from build123d import *

# Parameters (mm, degrees)
SKETCH_1_R      = 2.5
SKETCH_1_R_2    = 12.875
SKETCH_1_R_3    = 13.5
SKETCH_1_R_4    = 2
EXTRUDE_1_DEPTH = 5


with BuildPart() as part:
    # 草圖1 → 填料-伸長1 (new body)
    with BuildSketch(Plane.XY):
        with BuildLine():
            Line((-177.402767175, 46.597232825), (172.597232825, 46.597232825))
            Line((172.597232825, 46.597232825), (172.597232825, -3.218275341))
            Line((172.597232825, -3.218275341), (172.597232825, -12.212255112))
            ThreePointArc((172.597232825, -12.212255112), (171.299816564, -17.138210478), (167.744225572, -20.785962926))
            Line((167.744225572, -20.785962926), (157.766802923, -26.775637768))
            ThreePointArc((157.766802923, -26.775637768), (155.290289709, -27.838762374), (152.619810177, -28.201929955))
            Line((152.619810177, -28.201929955), (-158.204749101, -28.201929955))
            ThreePointArc((-158.204749101, -28.201929955), (-160.839127997, -27.848693549), (-163.287395186, -26.813939522))
            Line((-163.287395186, -26.813939522), (-172.48541326, -21.385442237))
            ThreePointArc((-172.48541326, -21.385442237), (-176.08684631, -17.731937443), (-177.402767175, -12.77343267))
            Line((-177.402767175, -12.77343267), (-177.402767175, -10.307650594))
            Line((-177.402767175, -10.307650594), (-177.402767175, -3.218275341))
            Line((-177.402767175, -3.218275341), (-177.402767175, 46.597232825))
        make_face()
        with Locations((118.590211239, 1.636058568)):
            Circle(SKETCH_1_R, mode=Mode.SUBTRACT)
        with Locations((154.590211239, 1.636058568)):
            Circle(SKETCH_1_R, mode=Mode.SUBTRACT)
        with Locations((136.590211239, 1.636058568)):
            Circle(SKETCH_1_R_2, mode=Mode.SUBTRACT)
        with Locations((-143.364629919, 1.616144457)):
            Circle(SKETCH_1_R_3, mode=Mode.SUBTRACT)
        with Locations((-130.636707858, 14.344066518)):
            Circle(SKETCH_1_R, mode=Mode.SUBTRACT)
        with Locations((-156.09255198, 14.344066518)):
            Circle(SKETCH_1_R, mode=Mode.SUBTRACT)
        with Locations((-130.636707858, -11.111777604)):
            Circle(SKETCH_1_R, mode=Mode.SUBTRACT)
        with Locations((-156.09255198, -11.111777604)):
            Circle(SKETCH_1_R, mode=Mode.SUBTRACT)
        with Locations((-152.402767175, 36.597232825)):
            Circle(SKETCH_1_R, mode=Mode.SUBTRACT)
        with Locations((-52.402767175, 36.597232825)):
            Circle(SKETCH_1_R, mode=Mode.SUBTRACT)
        with Locations((47.597232825, 36.597232825)):
            Circle(SKETCH_1_R, mode=Mode.SUBTRACT)
        with Locations((147.597232825, 36.597232825)):
            Circle(SKETCH_1_R, mode=Mode.SUBTRACT)
        with Locations((-161.364629919, 1.616144457)):
            Circle(SKETCH_1_R, mode=Mode.SUBTRACT)
        with Locations((-125.364629919, 1.616144457)):
            Circle(SKETCH_1_R, mode=Mode.SUBTRACT)
        with Locations((149.318133301, -11.091863493)):
            Circle(SKETCH_1_R, mode=Mode.SUBTRACT)
        with Locations((123.862289178, -11.091863493)):
            Circle(SKETCH_1_R, mode=Mode.SUBTRACT)
        with Locations((123.862289178, 14.363980629)):
            Circle(SKETCH_1_R, mode=Mode.SUBTRACT)
        with Locations((149.318133301, 14.363980629)):
            Circle(SKETCH_1_R, mode=Mode.SUBTRACT)
        with Locations((-46.268993965, 15.590754881)):
            Circle(SKETCH_1_R_4, mode=Mode.SUBTRACT)
        with Locations((-46.268993965, -14.409245119)):
            Circle(SKETCH_1_R_4, mode=Mode.SUBTRACT)
        with Locations((43.737437285, 15.590754881)):
            Circle(SKETCH_1_R_4, mode=Mode.SUBTRACT)
        with Locations((43.737437285, -14.409245119)):
            Circle(SKETCH_1_R_4, mode=Mode.SUBTRACT)
    extrude(amount=EXTRUDE_1_DEPTH)


solid = part.part
Here's how the part is built. I have some questions about the finished solid (model axes, mm). Coordinates: 2 decimals unless noted, no trailing zeros. Answer as CSV lines item,"result".
Item 1: Imagine slicing it at A-A on z = 3.5. Give the number of separate pieces and of enclosed holes in the cut face, plus the area to 3 significant figures.
Results found:
separate pieces,"1"
enclosed holes,"22"
area,"24,500 mm2"
Item 2: We'd pull the mould along Y, two halves only. Please class faces 1 (the face through (162.825, -23.739, 2.465)), 2 (the face through (-156.85, 2.21, 2.46)), 3 (the face through (0, 10, 5)): +Y half, -Y half, draft (parallel to the pull), parting line (faces both ways), or undercut.
Results found:
face 1,"-Y half"
face 2,"undercut"
face 3,"draft"
Item 3: If I drill on line 1 (X direction, y = 36, z = 1.2); line 2 (X direction, y = -1.5, z = 1.3); line 3 (X direction, y = -14.5, z = 4.5), over which ranges is the centre line in solid material (lowest first)?
Results found:
line 1,"-177.4 to -154.83, -149.98 to -54.83, -49.98 to 45.17, 50.02 to 145.17, 150.02 to 172.6"
line 2,"-177.4 to -156.5, -130.23 to 124.1, 149.08 to 172.6"
line 3,"-177.25 to -48.27, -44.27 to 41.74, 45.74 to 172.33"
Item 4: For pin 1 (8 mm diameter, centred on x = 123.86, y = 14.36, fed in from -Z), with a flat end and sliding along its axis, tell me the tip position at first contact or that it passes through.
Results found:
pin 1,"z = 0"
